Here's how the part is built. I have some questions about the finished solid (model axes, mm). A direction names the side the tool comes from. Give positions to 0.01 mm unless a question says otherwise; leave off trailing zeros. Loops run counter-clockwise (first coordinate to the right, second up) from the corner with the lowest first, then second, coordinate; pieces in that order, holes last. Notation, with made-up numbers: M -12.5,2 L 28.5,2 A18 cw 28.5,17 Z; hole C 6.25,51.5 d3. An arc over 180 degrees is marked long. Answer as CSV lines item,"result". Start each with the question number.
Item 1: I want a section at C-C on z = -11. List the corners of the cut face in (x, y) for me, plus the area to 3 significant figures.
Item 2: I want a section at A-A on x = 2.25. List the corners of the cut face in (y, z) for me, plus the area to 3 significant figures.
Item 3: I want a section at D-D on x = 20. List the corners of the cut face in (y, z) for me, plus the area to 3 significant figures.
Item 4: Will these pins go through, and if not, where does the flat tip stop? P1, Ø2.5, axis at x = 22.5, z = 33, coming from the -Y side; P2, Ø15, axis at x = 50.5, z = 14, coming from the -Y side; P3, Ø5, axis at y = -13, z = 24.8, coming from the -X side; P4, Ø5, axis at x = -1.5, z = 14.5, coming from the -Y side.
Item 5: If we mould it in two halves opening along X, with no side actions, what happens to faces 6 (the flat face through (67, 11, 11)), 7 (the flat face through (5, -1, 2)), 8 (the flat face through (-22, 5, 11)), 9 (the flat face through (18, 13, 20))? For each: released by +X, released by -X, zero draft, split by the parting line, or undercut.
Item 6: For faces 1 (the flat face through (18, 6, 29.655)), 2 (the cylindrical face through (-27.696, 19.465, 10.962)), 3 (the flat face through (52, 11, -14.3)), 4 (the flat face through (-22, 11, -14.3)), 5 (the flat face through (18, 13, -19.5)), which set-ups out of +Z, -Z, +X, -X, +Y, -Y let a thin tool reach every point of the face, with its end or its side?
Item 7: I want a section at B-B on z = 11.1. List the corners of the cut face in (x, y) for me.
Item 8: If I drill on line 1 along Y through (x, z) = (3.85, -24.2); line 2 along Y through (x, z) = (-35.5, 0); line 3 along X through (y, z) = (-13, -17.5), over which ranges is the centre line in solid material (lowest first)? Write a range as from..to.
from build123d import *

# Parameters (mm, degrees)
SKETCH3_W            = 57
SKETCH3_H            = 34
SKETCH3_R            = 2.2
BOSS_EXTRUDE2_DEPTH  = 5
BOSS_EXTRUDE3_DEPTH  = 32
SKETCH5_R            = 6.9
CUT_EXTRUDE1_DEPTH   = 19
BOSS_EXTRUDE4_DEPTH  = 8
SKETCH7_W            = 6
SKETCH7_H            = 4.5
BOSS_EXTRUDE5_DEPTH  = 39.5
BOSS_EXTRUDE6_DEPTH  = 32
BOSS_EXTRUDE7_DEPTH  = 32
SKETCH11_W           = 6
SKETCH11_H           = 8.410531804
BOSS_EXTRUDE8_DEPTH  = 58.155109
SKETCH12_W           = 6
SKETCH12_H           = 1.5
BOSS_EXTRUDE9_DEPTH  = 9
SKETCH13_W           = 50.8
SKETCH13_H           = 12
BOSS_EXTRUDE10_DEPTH = 30
SKETCH14_W           = 50.8
SKETCH14_H           = 12
BOSS_EXTRUDE11_DEPTH = 44.75
SKETCH15_R           = 3
SKETCH15_R_2         = 3.129089935
BOSS_EXTRUDE12_DEPTH = 5


with BuildPart() as part:
    # Sketch3 → Boss-Extrude2 (new body)
    with BuildSketch(Plane(origin=(0, 0, 0), x_dir=(0, 0, -1), z_dir=(1, 0, 0))):
        Rectangle(SKETCH3_W, SKETCH3_H)
        with Locations((-24.8, -3.1)):
            Circle(SKETCH3_R, mode=Mode.SUBTRACT)
        with Locations((-24.8, -13)):
            Circle(SKETCH3_R, mode=Mode.SUBTRACT)
        with Locations((24.2, -3.1)):
            Circle(SKETCH3_R, mode=Mode.SUBTRACT)
        with Locations((24.2, -13)):
            Circle(SKETCH3_R, mode=Mode.SUBTRACT)
    extrude(amount=BOSS_EXTRUDE2_DEPTH)

    # Sketch4 → Boss-Extrude3 (add)
    with BuildSketch(Plane(origin=(5, 0, 0), x_dir=(0, 0, -1), z_dir=(1, 0, 0))):
        Polygon((-28.5, 17), (12, 17), (12, 15), (-20, 15), (-20, 10.5), (-28.5, 10.5), align=None)
    extrude(amount=BOSS_EXTRUDE3_DEPTH)

    # Sketch5 → Cut-Extrude1 (cut)
    with BuildSketch(Plane(origin=(0, 17, 0), x_dir=(1, 0, 0), z_dir=(0, 1, 0))):
        with Locations((20, -11.1)):
            Circle(SKETCH5_R)
    extrude(amount=-CUT_EXTRUDE1_DEPTH, mode=Mode.SUBTRACT)

    # Sketch6 → Boss-Extrude4 (add)
    with BuildSketch(Plane.XY.offset(28.5)):
        Polygon((0, 17), (37, 17), (37, 10.5), (5, 10.5), (5, -5.696050601), (0, -5.696050601), align=None)
    extrude(amount=BOSS_EXTRUDE4_DEPTH)

    # Sketch7 → Boss-Extrude5 (add)
    with BuildSketch(Plane(origin=(0, 0, 20), x_dir=(-1, 0, 0), z_dir=(0, 0, -1))):
        with Locations((-34, 12.75)):
            Rectangle(SKETCH7_W, SKETCH7_H)
    extrude(amount=BOSS_EXTRUDE5_DEPTH)

    # Sketch8 → Boss-Extrude6 (add)
    with BuildSketch(Plane(origin=(5, 0, 0), x_dir=(0, 0, -1), z_dir=(1, 0, 0))):
        Polygon((-36.5, -5.696050601), (-32.171374704, -5.696050601), (-32.171374704, 2.089468196), (-29.655108528, 2.089468196), (-29.655108528, 10.5), (-32.171374704, 10.5), (-36.5, 10.5), align=None)
    extrude(amount=BOSS_EXTRUDE6_DEPTH)

    # Sketch9 → Boss-Extrude7 (add)
    with BuildSketch(Plane(origin=(5, 0, 0), x_dir=(0, 0, -1), z_dir=(1, 0, 0))):
        Polygon((12, 17), (28.5, 17), (28.5, 12), (19.5, 12), (19.5, 15), (12, 15), align=None)
    extrude(amount=BOSS_EXTRUDE7_DEPTH)

    # Sketch11 → Boss-Extrude8 (add)
    with BuildSketch(Plane(origin=(0, 0, 29.655108528), x_dir=(-1, 0, 0), z_dir=(0, 0, -1))):
        with Locations((-34, 6.294734098)):
            Rectangle(SKETCH11_W, SKETCH11_H)
    extrude(amount=BOSS_EXTRUDE8_DEPTH)

    # Sketch12 → Boss-Extrude9 (add)
    with BuildSketch(Plane(origin=(0, 0, -19.5), x_dir=(-1, 0, 0), z_dir=(0, 0, -1))):
        with Locations((-34, 11.25)):
            Rectangle(SKETCH12_W, SKETCH12_H)
    extrude(amount=BOSS_EXTRUDE9_DEPTH)

    # Sketch13 → Boss-Extrude10 (add)
    with BuildSketch(Plane(origin=(37, 0, 0), x_dir=(0, 0, -1), z_dir=(1, 0, 0))):
        with Locations((-11.1, 11)):
            Rectangle(SKETCH13_W, SKETCH13_H)
    extrude(amount=BOSS_EXTRUDE10_DEPTH)

    # Sketch14 → Boss-Extrude11 (add)
    with BuildSketch(Plane.ZY):
        with Locations((11.1, 11)):
            Rectangle(SKETCH14_W, SKETCH14_H)
    extrude(amount=BOSS_EXTRUDE11_DEPTH)

    # Sketch15 → Boss-Extrude12 (add)
    with BuildSketch(Plane(origin=(0, 17, 0), x_dir=(1, 0, 0), z_dir=(0, 1, 0))):
        with Locations((2.25, -11.1)):
            Circle(SKETCH15_R)
        with Locations((46.82, -11.1)):
            Circle(SKETCH15_R)
        with Locations((-24.57, -11.1)):
            Circle(SKETCH15_R_2)
    extrude(amount=BOSS_EXTRUDE12_DEPTH)


solid = part.part
Result:
1,outline,"M -44.75,5 L 0,5 L 0,-17 L 5,-17 L 5,15 L 31,15 L 31,2.09 L 37,2.09 L 37,5 L 67,5 L 67,17 L -44.75,17 Z"
1,area,"1,210 mm^2"
2,outline,"M -17,-28.5 L 17,-28.5 L 17,8.1 L 22,8.1 L 22,14.1 L 17,14.1 L 17,36.5 L -5.7,36.5 L -5.7,28.5 L -17,28.5 Z; hole C -13,-24.2 d4.4; hole C -13,24.8 d4.4; hole C -3.1,-24.2 d4.4; hole C -3.1,24.8 d4.4"
2,area,"2,090 mm^2"
3,outline,"M -5.7,32.17 L 2.09,32.17 L 2.09,29.66 L 10.5,29.66 L 10.5,20 L 15,20 L 15,18 L 17,18 L 17,36.5 L -5.7,36.5 Z; M 12,-28.5 L 17,-28.5 L 17,4.2 L 15,4.2 L 15,-19.5 L 12,-19.5 Z"
3,area,"295 mm^2"
4,P1,"y = -5.7"
4,P2,"y = 5"
4,P3,"x = 0"
4,P4,"y = -17"
5,face 6,"released by +X"
5,face 7,"undercut"
5,face 8,"zero draft"
5,face 9,"undercut"
6,face 1,"-Z, -Y"
6,face 2,"+Y"
6,face 3,"-Z, +X, +Y, -Y"
6,face 4,"-Z, -X, +Y, -Y"
6,face 5,"-Y"
7,outline,"M -44.75,5 L 0,5 L 0,-17 L 5,-17 L 5,15 L 13.1,15 L 13.1,17 L 5.25,17 L 5.25,22 L -0.75,22 L -0.75,17 L -21.44,17 L -21.44,22 L -27.7,22 L -27.7,17 L -44.75,17 Z; M 26.9,15 L 31,15 L 31,2.09 L 37,2.09 L 37,5 L 67,5 L 67,17 L 49.82,17 L 49.82,22 L 43.82,22 L 43.82,17 L 26.9,17 Z"
8,line 1,"-17..-15.2, -10.8..-5.3, -0.9..17"
8,line 2,"5..17"
8,line 3,"0..5"
